Job drawing, mm, ordinate dimensions from the low corner. One solid piece. A direction names the side the tool comes from. Coordinates: 2 decimals unless noted, no trailing zeros. Write each loop counter-clockwise with the first axis right and the second up, starting at its lowest first coordinate (ties: lowest second). Pieces come first, ordered by that corner, then holes.
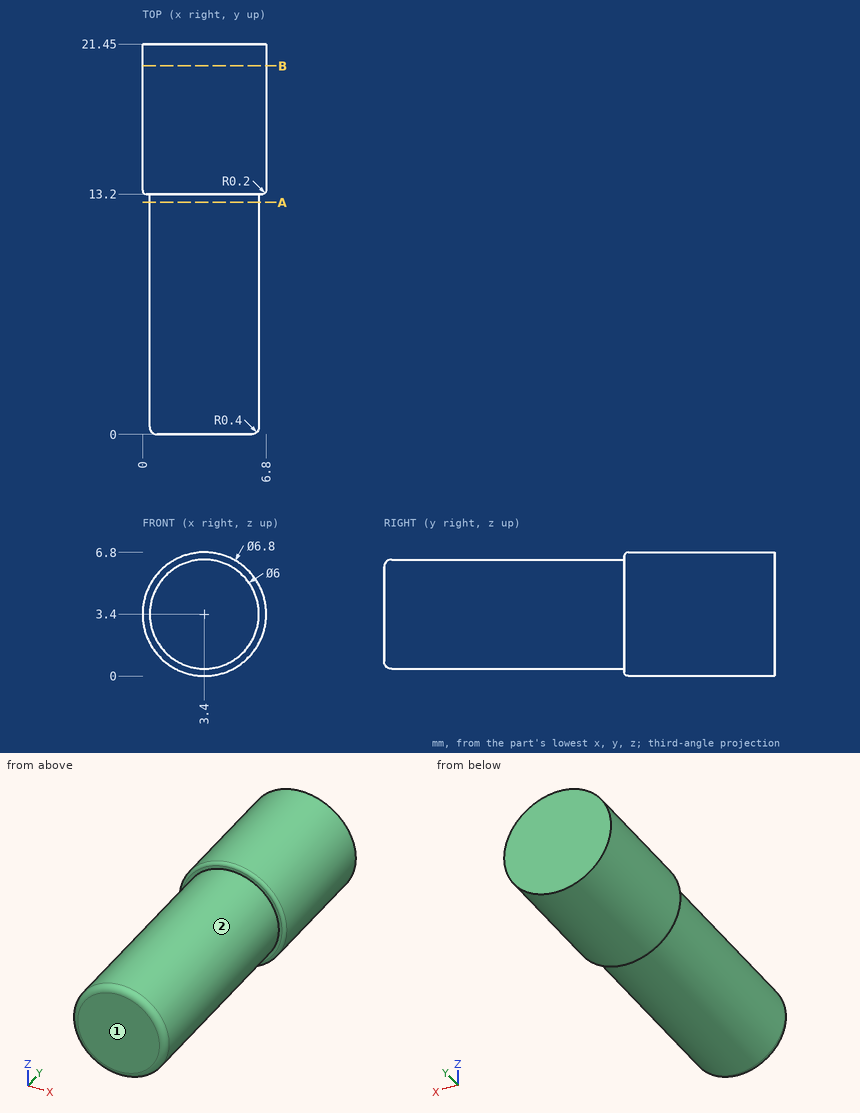
1. Saw through at B-B on y = 20.25. List the corners of the cut face in (x, z).
Computed values:
outline: circle Ø6.8 at (3.4, 3.4)
2. Saw through at A-A on y = 12.75. List the corners of the cut face in (x, z).
Computed values:
outline: circle Ø6 at (3.4, 3.4)
3. Probe line 1 along X through (y, z) = (18.75, 2.25); line 2 along Z through (x, y) = (3.5, 11.25); line 3 along Y through (x, z) = (5, 5.5). List the from-to ranges inside material, lowest first.
Computed values:
line 1: x = 0.2 to 6.6
line 2: z = 0.4 to 6.4
line 3: y = 0 to 21.45
4. 3-axis set-ups, long thin cutter, end or side, ignore diameter. For the marked faces 1 and 2: which of +Z, -Z, +X, -X, +Y, -Y reach the whole face in a straight line?
Computed values:
face 1: +Z, -Z, +X, -X, -Y
face 2: -Y
5. Flat gauge pins, fed straight in: pin 1 (2 mm diameter, centred on y = 6.5, z = 4, fed in from +X); pin 2 (1 mm diameter, centred on x = 1.5, y = 6, fed in from +Z). Where does each tip first touch, or does it go through?
Computed values:
pin 1: stops at x = 6.4
pin 2: stops at z = 6.05
